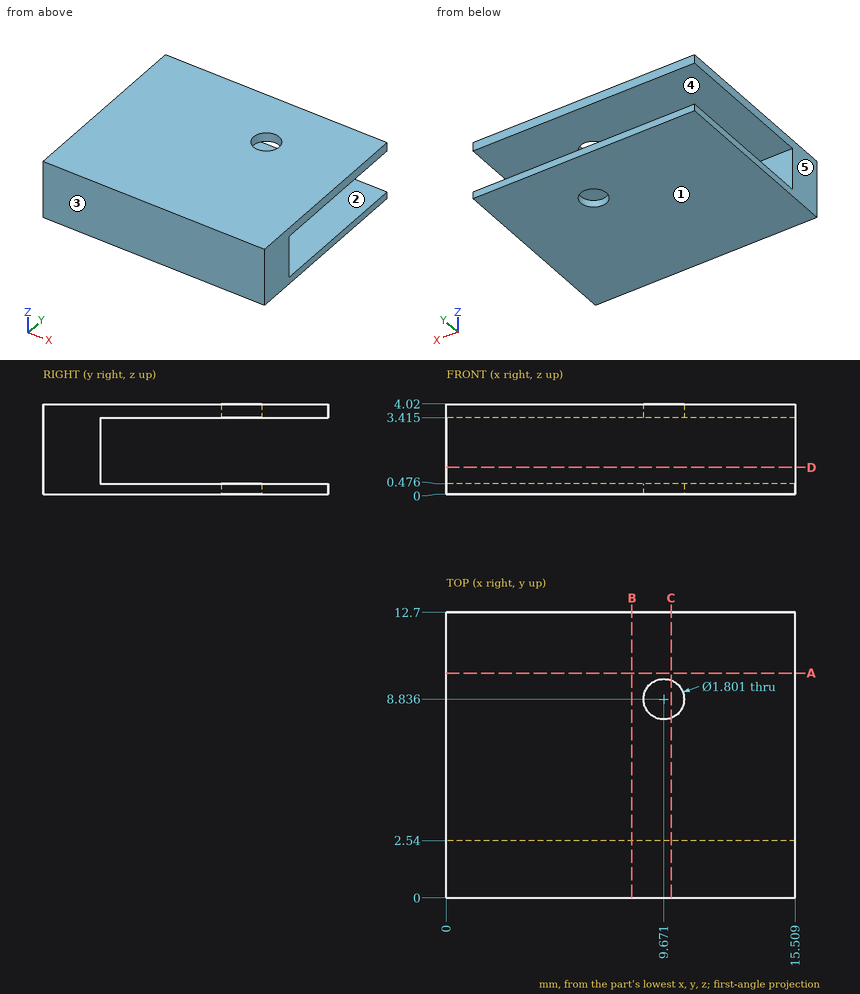
Input: dimensioned drawing with shaded views. Units: mm. Origin: part minimum x, y, z. A direction names the side the tool comes from. Give positions to 0.01 mm unless a question says otherwise; leave off trailing zeros. Write each loop counter-clockwise with the first axis right and the second up, starting at its lowest first coordinate (ties: lowest second). Pieces come first, ordered by that corner, then holes. Notation, with made-up numbers: (71, 24.5) - (104, 24.5) arc R17 ccw to (104, 37.5) - close; hole circle Ø9 at (-9.5, 60). An arc over 180 degrees is marked (long way). Write item = value, one per line. Start each with the question number.
1) Cut plane C-C (x = 10). Return loops of the section in (y, z) (1 decimal).
2) Cut plane D-D (z = 1.2). Return loops of the section in (x, y).
3) Reachability of the marked faces 4 and 5 from +Z, -Z, +X, -X, +Y, -Y: full face, straight path, thin tool, end or side. Return the list, or none.
4) Material intervals for L1, parallel to Z at x = 3.75, y = 8.25 (1 decimal); L2, parallel to Y at x = 1.75, z = 2.2, sorted ascending. Write a range as [from, to].
5) Draft query along Z for the marked faces 1, 2 and 3. Return one class per face: pulls with the +Z half, pulls with the -Z half, needs draft (parallel to the pull), parting line crosses it, or undercut.
6) Cut plane A-A (y = 10). Return loops of the section in (x, z) (1 decimal).
7) Cut plane B-B (x = 8.25). Return loops of the section in (y, z) (1 decimal).
Answers follow:
q1.outline = (0, 0) - (8, 0) - (8, 0.5) - (2.5, 0.5) - (2.5, 3.4) - (8, 3.4) - (8, 4) - (0, 4) - close; (9.7, 0) - (12.7, 0) - (12.7, 0.5) - (9.7, 0.5) - close; (9.7, 3.4) - (12.7, 3.4) - (12.7, 4) - (9.7, 4) - close
q2.outline = (0, 0) - (15.51, 0) - (15.51, 2.54) - (0, 2.54) - close
q3.face_4 = +X, -X, +Y
q3.face_5 = +Z, -Z, -X, +Y, -Y
q4.L1 = [0, 0.5], [3.4, 4]
q4.L2 = [0, 2.54]
q5.face_1 = pulls with the -Z half
q5.face_2 = undercut
q5.face_3 = needs draft
q6.outline = (0, 0) - (15.5, 0) - (15.5, 0.5) - (0, 0.5) - close; (0, 3.4) - (15.5, 3.4) - (15.5, 4) - (0, 4) - close
q7.outline = (0, 0) - (12.7, 0) - (12.7, 0.5) - (2.5, 0.5) - (2.5, 3.4) - (12.7, 3.4) - (12.7, 4) - (0, 4) - close
